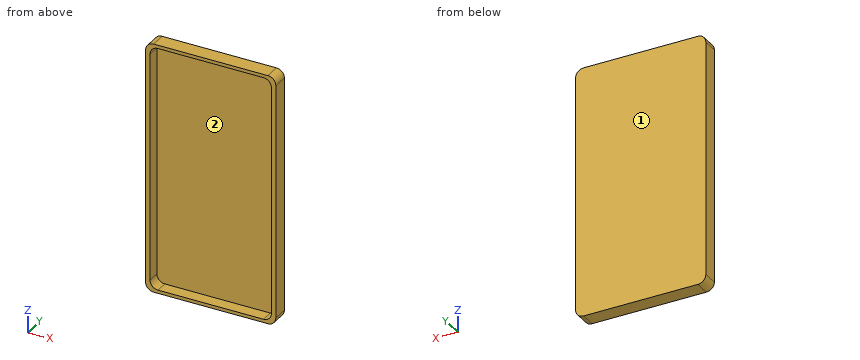
from build123d import *

# Parameters (mm, degrees)
F0_W     = 83
F0_H     = 160
F0_W_2   = 77.461682
F0_H_2   = 155.82101
F1_DEPTH = 9.906
F2_DEPTH = 2
F3_R     = 5.08


with BuildPart() as f1:
    # F0 (on Front) → F1 (new body)
    with BuildSketch(Plane.XZ):
        Rectangle(F0_W, F0_H)
        Rectangle(F0_W_2, F0_H_2, mode=Mode.SUBTRACT)
    extrude(amount=F1_DEPTH)

    # F0 (on Front) → F2 (join)
    with BuildSketch(Plane.XZ):
        Rectangle(F0_W_2, F0_H_2)
    extrude(amount=F2_DEPTH)

    # F3
    f3_edges = [f1.edges().sort_by_distance(p)[0] for p in [
        (-38.730841, -5.953, 77.910505),
        (38.730841, -5.953, 77.910505),
        (-38.730841, -5.953, -77.910505),
        (38.730841, -5.953, -77.910505),
        (41.5, -4.953, -80),
        (-41.5, -4.953, 80),
        (-41.5, -4.953, -80),
        (41.5, -4.953, 80),
    ]]
    fillet(f3_edges, radius=F3_R)


solid = f1.part
Part model, mm, in its own coordinate system. Face numbers are marked on the shaded views. Coordinates: 2 decimals unless noted, no trailing zeros. Order: outer loops, then holes, each group sorted by start corner. A loop starts at its lowest first (then second) coordinate and runs counter-clockwise, first axis right, second up.
(1) Slice it at C-C, the plane z = -12. Write the cut outline in (x, y), and give its area (3 significant figures).
Check sheet entries:
outline: (-41.5, -9.91) - (-38.73, -9.91) - (-38.73, -2) - (38.73, -2) - (38.73, -9.91) - (41.5, -9.91) - (41.5, 0) - (-41.5, 0) - close
area: 210 mm2
(2) Slice it at B-B, the plane x = -9.5. Write the cut outline in (y, z), and give its area (3 significant figures).
Check sheet entries:
outline: (-9.91, -80) - (0, -80) - (0, 80) - (-9.91, 80) - (-9.91, 77.91) - (-2, 77.91) - (-2, -77.91) - (-9.91, -77.91) - close
area: 353 mm2
(3) Pin check, flat tip, straight feed: pin 1 Ø2 at (x, z) = (10.5, 8.5) entering from -Y. Stop position of the tip, or through.
Check sheet entries:
pin 1: stops at y = -2
(4) Pull direction Z, two halves, no side cores. Call the marked faces 1 and 2: pulls with the +Z half, pulls with the -Z half, needs draft (parallel to the pull), parting line crosses it, or undercut.
Check sheet entries:
face 1: needs draft
face 2: undercut
(5) Slice it at A-A, the plane y = -6. Write the cut outline in (x, z), and give its area (3 significant figures).
Check sheet entries:
outline: (-41.5, -74.92) arc R5.08 ccw to (-36.42, -80) - (36.42, -80) arc R5.08 ccw to (41.5, -74.92) - (41.5, 74.92) arc R5.08 ccw to (36.42, 80) - (-36.42, 80) arc R5.08 ccw to (-41.5, 74.92) - close; hole (-38.73, -72.83) arc R5.08 ccw to (-33.65, -77.91) - (33.65, -77.91) arc R5.08 ccw to (38.73, -72.83) - (38.73, 72.83) arc R5.08 ccw to (33.65, 77.91) - (-33.65, 77.91) arc R5.08 ccw to (-38.73, 72.83) - close
area: 1,210 mm2
(6) Probe L1, parallel to Z at x = 27.5, y = -3.25; L2, parallel to X at y = -8, z = -50; L3, parallel to Y at x = 31, z = -44. List the from-to ranges inside material, lowest first.
Check sheet entries:
L1: z = -80 to -77.91, 77.91 to 80
L2: x = -41.5 to -38.73, 38.73 to 41.5
L3: y = -2 to 0
